CAD build for the part. Positions are in the model's coordinates, mm. Coordinates: 2 decimals unless noted, no trailing zeros. Loops run counter-clockwise (first coordinate to the right, second up) from the corner with the lowest first, then second, coordinate; pieces in that order, holes last. Notation, with made-up numbers: (57, 46) -> (97, 46) arc R28 ccw to (97, 78) -> close; hole circle Ø9 at (19.5, 68.5). An arc over 180 degrees is marked (long way). Write each question's results on one line, items separated by ' | '.
```python
from build123d import *

# Parameters (mm, degrees)
F0_R     = 26
F0_R_2   = 24
F0_R_3   = 22
F0_R_4   = 20
F1_DEPTH = 3.5
F2_DEPTH = 3.25
F3_SIZE  = 0.3


with BuildPart() as f1:
    # F0 (on Front) → F1 (new body, symmetric)
    with BuildSketch(Plane.XZ):
        Circle(F0_R)
        Circle(F0_R_2, mode=Mode.SUBTRACT)
        Circle(F0_R_3)
        Circle(F0_R_4, mode=Mode.SUBTRACT)
    extrude(amount=F1_DEPTH, both=True)

    # F0 (on Front) → F2 (join, symmetric)
    with BuildSketch(Plane.XZ):
        Circle(F0_R_2)
        Circle(F0_R_3, mode=Mode.SUBTRACT)
    extrude(amount=F2_DEPTH, both=True)

    # F3
    f3_edges = [f1.edges().sort_by_distance(p)[0] for p in [
        (-26, -3.5, 0),
        (-26, 3.5, 0),
        (-20, -3.5, 0),
        (-20, 3.5, 0),
    ]]
    chamfer(f3_edges, length=F3_SIZE)


solid = f1.part
```
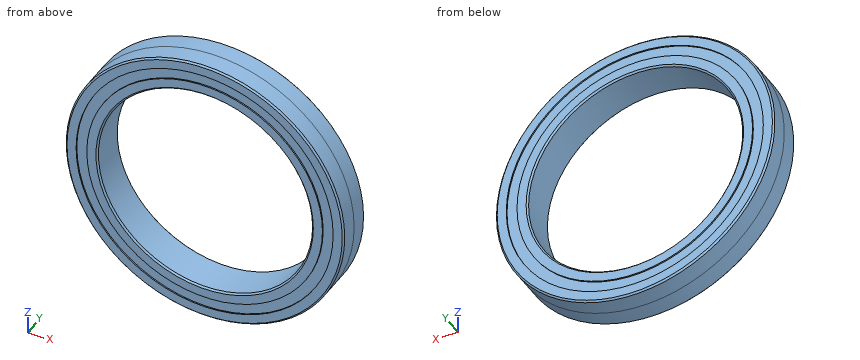
Q1. Cut at C-C on y = 2.5. Write the cut outline in (x, z).
Results are:
outline: circle Ø52 at (0, 0); hole circle Ø40 at (0, 0)
Q2. Wall check: L1, parallel to Z at x = 0, y = -0.25; L2, parallel to Z at x = 0, y = -3.35; L3, parallel to Z at x = 0, y = 3.45. Give the ranges that are in metal, low to high. Write a range as from..to.
Results are:
L1: -26..-20, 20..26 | L2: -25.85..-24, -22..-20.15, 20.15..22, 24..25.85 | L3: -25.75..-24, -22..-20.25, 20.25..22, 24..25.75
Q3. Drop flat-ended pins along their axis: pin 1 (4 mm diameter, centred on x = -15.5, y = -1.5, fed in from +Z); pin 2 (1.5 mm diameter, centred on y = 2.5, z = -17, fed in from +X). Give the stop position or say it passes through.
Results are:
pin 1: z = 22.22 | pin 2: x = 20.3
